Can you work these out from the model? Positions are in its coordinate system, mm. A direction names the side the tool comes from. Round coordinates to 2 decimals unless told otherwise and drop trailing zeros. Loops run counter-clockwise (first coordinate to the right, second up) from the corner with the lowest first, then second, coordinate; pieces in that order, holes last. Notation, with made-up numbers: (81, 6.25) - (107, 6.25) arc R9 cw to (107, 19.25) - close; hole circle Ø2 at (50.5, -5.5). An arc over 180 degrees is marked (long way). Answer as CSV lines item,"result".
```python
from build123d import *

# Parameters (mm, degrees)
F0_R        = 1.55
F1_DEPTH    = 2
F2_W        = 5.8800544143
F2_H        = 19.6606332908
F2_W_2      = 2
F3_DEPTH    = 2
F4_T1_DEPTH = 39.6606332908


# Not quite as in the source:
# - a fillet or chamfer that OpenCascade refuses, or shapes differently, is made with other operations: its cross-section is extruded or revolved along the edge and cut away or added


with BuildPart() as f1:
    # F0 (on Right) → F1 (new body)
    with BuildSketch(Plane.YZ):
        with BuildLine():
            Line((-14.6106332908, -3), (-13.2183143869, -3))
            Line((-13.2183143869, -3), (5.05, -3))
            Line((5.05, -3), (5.05, 5.273589902))
            Line((5.05, 5.273589902), (3.9867715302, 7.2948440555))
            ThreePointArc((3.9867715302, 7.2948440555), (1.9828252763, 9.159944049), (-0.7469684056, 9.3664023457))
            Line((-0.7469684056, 9.3664023457), (-11.3228132649, 6.5356446488))
            Line((-11.3228132649, 6.5356446488), (-16.7690545021, 2.0835589443))
            ThreePointArc((-16.7690545021, 2.0835589443), (-17.372034822, -1.1724596298), (-14.6106332908, -3))
        make_face()
        with Locations((-12.5, 0.9715808555)):
            Circle(F0_R, mode=Mode.SUBTRACT)
        Circle(F0_R, mode=Mode.SUBTRACT)
        with Locations((-6, 5)):
            Circle(F0_R, mode=Mode.SUBTRACT)
        with Locations((0, 5)):
            Circle(F0_R, mode=Mode.SUBTRACT)
    extrude(amount=F1_DEPTH)

    # F2 (on face) → F3 (join)
    with BuildSketch(Plane(origin=(0, 0, -3), x_dir=(1, 0, 0), z_dir=(0, 0, -1))):
        with Locations((4.9400272071, 4.7803166454)):
            Rectangle(F2_W, F2_H)
        with Locations((1, 4.7803166454)):
            Rectangle(F2_W_2, F2_H)
    extrude(amount=F3_DEPTH)

    # F4: fillet of radius 4 on 1 edges, made by hand

    # F4_s2 → F4_t1 (cut)
    with BuildSketch(Plane.XZ.offset(-15.05)):
        with BuildLine():
            ThreePointArc((4, -5), (1.1715728753, -3.8284271247), (0, -1))
            Line((0, -1), (0, -5))
            Line((0, -5), (4, -5))
        make_face()
    extrude(amount=F4_T1_DEPTH, mode=Mode.SUBTRACT)


solid = f1.part
```
Q1. Imagine slicing it at C-C (y = 0). Write out the boundary of the cut face in (x, z), then the cut area to 3 significant figures.
Checks:
outline,"(0, 1.55) - (2, 1.55) - (2, 3.45) - (0, 3.45) - close; (0, 6.55) - (2, 6.55) - (2, 9.49) - (0, 9.49) - close; (0.04, -1.55) arc R4 ccw to (4, -5) - (7.88, -5) - (7.88, -3) - (2, -3) - (2, -1.55) - close"
area,"24.9 mm²"
Q2. If I drill on line 1 along Z through (x, y) = (1.55, 0); line 2 along X through (y, z) = (3.5, 2.5); line 3 along Z through (x, y) = (5.25, -9.5), over which ranges is the centre line in solid material (lowest first)? Write a range as [from, to].
Checks:
line 1,"[-4.16, -1.55], [1.55, 3.45], [6.55, 9.49]"
line 2,"[0, 2]"
line 3,"[-5, -3]"
Q3. Imagine slicing it at B-B (z = 3.75). Write out the boundary of the cut face in (x, y), then the cut area to 3 significant figures.
Checks:
outline,"(0, -14.73) - (2, -14.73) - (2, -6.92) - (0, -6.92) - close; (0, -5.08) - (2, -5.08) - (2, -0.92) - (0, -0.92) - close; (0, 0.92) - (2, 0.92) - (2, 5.05) - (0, 5.05) - close"
area,"32.2 mm²"
Q4. I'm going to push flat-ended pins straight in: pin 1 Ø6.5 at (y, z) = (-10.5, 3) entering from +X; pin 2 Ø2 at (x, z) = (1.5, 4.5) entering from -Y; pin 3 Ø6 at (y, z) = (-7.5, 4.5) entering from -X; pin 4 Ø3 at (x, y) = (5, -6.5) entering from +Z. Where does each tip first touch, or does it pass through?
Checks:
pin 1,"x = 2"
pin 2,"y = -15.04"
pin 3,"x = 0"
pin 4,"z = -3"
Q5. Imagine slicing it at A-A (y = -6). Write out the boundary of the cut face in (x, z), then the cut area to 3 significant figures.
Checks:
outline,"(0, -1) arc R4 ccw to (4, -5) - (7.88, -5) - (7.88, -3) - (2, -3) - (2, 3.45) - (0, 3.45) - close; (0, 6.55) - (2, 6.55) - (2, 7.96) - (0, 7.96) - close"
area,"28.0 mm²"
Q6. We'd pull the mould along Y, two halves only. Please class faces 4 (the flat face through (6, -5, -5)), 5 (the flat face through (0.986, 4.526, 6.27)), 6 (the cylindrical face through (0.99, -7.55, 5.07)): pulls with the +Y half, pulls with the -Y half, needs draft (parallel to the pull), parting line crosses it, or undercut.
Checks:
face 4,"needs draft"
face 5,"pulls with the +Y half"
face 6,"undercut"
Q7. On a 3-axis mill with a long thin cutter (end or side, diameter ignored), from which of +Z, -Z, +X, -X, +Y, -Y can I reach the whole of each face in a straight line? I mean faces 1 (the flat face through (5, -5, -3)), 2 (the flat face through (0.99, -5.96, 7.97)), 3 (the flat face through (4, -14.611, -4)). Say none if no direction works.
Checks:
face 1,"+Z, +X, +Y, -Y"
face 2,"+Z, +X, -X, -Y"
face 3,"-Z, +X, -X, -Y"
Q8. Imagine slicing it at D-D (x = 1.5). Write out the boundary of the cut face in (y, z).
Checks:
outline,"(-16.77, 2.08) arc R3 ccw to (-14.61, -3) - (-14.61, -4.12) - (5.05, -4.12) - (5.05, 5.27) - (3.99, 7.29) arc R4.14 ccw to (-0.75, 9.37) - (-11.32, 6.54) - close; hole circle Ø3.1 at (-12.5, 0.97); hole circle Ø3.1 at (-6, 5); hole circle Ø3.1 at (0, 0); hole circle Ø3.1 at (0, 5)"
